Here's how the part is built. I have some questions about the finished solid (model axes, mm). Coordinates: 2 decimals unless noted, no trailing zeros. Write each loop counter-clockwise with the first axis right and the second up, starting at its lowest first coordinate (ties: lowest second). Pieces come first, ordered by that corner, then holes. Notation, with made-up numbers: (82, -29) - (130, -29) arc R14 ccw to (130, -24) - close; hole circle Ø2 at (39.25, 64.5). An arc over 180 degrees is marked (long way). Answer in a Markdown table with one row per item. Add a question column.
Item 1: Imagine slicing it at D-D (x = 134.5). Please give me the cut outline in (y, z).
Item 2: If I drill on probe 1 along Y at (x, z) = (118.5, 63); probe 2 along X at (y, z) = (-15, 8.5); probe 3 along Z at (x, y) = (-47, -74.5), over which ranges is the centre line in solid material (lowest first)? Write a range as from..to.
Item 3: Imagine slicing it at C-C (z = 71.5). Please give me the cut outline in (x, y).
Item 4: Imagine slicing it at B-B (y = -29.5). Please give me the cut outline in (x, z).
Item 5: I'm going to push flat-ended pins straight in: pin 1 (4 mm diameter, centred on y = -114, z = -4.5, fed in from -X); pin 2 (10 mm diameter, centred on y = -34.5, z = 7, fed in from -X); pin 3 (3 mm diameter, centred on x = -71.5, z = -162.5, fed in from +Y). Where does each tip first touch, or does it pass through?
Item 6: Imagine slicing it at A-A (x = 2). Please give me the cut outline in (y, z).
from build123d import *

# Parameters (mm, degrees)
F1_DEPTH = 139.7
F3_DEPTH = 254


with BuildPart() as f1:
    # F0 (on Front) → F1 (new body)
    with BuildSketch(Plane.XZ):
        Polygon((-101.6, 100.334205), (-152.4, 12.7), (-101.6, -140.965795), (-93.98, -204.465795), (0, -204.465795), (0, 100.334205), align=None)
        Polygon((101.6, 100.334205), (0, 100.334205), (0, -204.465795), (93.98, -204.465795), (101.6, -140.965795), (152.4, 12.7), align=None)
    extrude(amount=F1_DEPTH)

    # F2 (on Right) → F3 (cut, symmetric)
    with BuildSketch(Plane.YZ):
        Polygon((11.297926, 100.633033), (-45.92489, 100.633033), (0, 12.690174), (-88.975355, -204.561785), (-139.714777, -28.677866), (-46.015032, 100.633033), (-152.156293, 100.633033), (-152.156293, -218.677998), (11.297926, -218.677998), align=None)
    extrude(amount=F3_DEPTH, both=True, mode=Mode.SUBTRACT)


solid = f1.part
Here are the results:
| question | item | result |
|---|---|---|
| 1 | outline | (-139.7, -28.73) - (-136.03, -41.45) - (-22.17, -41.45) - (0, 12.69) - (-16.13, 43.58) - (-87.36, 43.58) - (-139.7, -28.66) - close |
| 2 | probe 1 | y = -73.28..-26.27 |
| 2 | probe 2 | x = -151.01..151.01 |
| 2 | probe 3 | z = -169.22..61.32 |
| 3 | outline | (-118.31, -67.13) - (118.31, -67.13) - (118.31, -30.71) - (-118.31, -30.71) - close |
| 4 | outline | (-152.4, 12.7) - (-128.58, -59.34) - (128.58, -59.34) - (152.4, 12.7) - (119.66, 69.18) - (-119.66, 69.18) - close |
| 5 | pin 1 | stops at x = -147.38 |
| 5 | pin 2 | stops at x = -152.17 |
| 5 | pin 3 | stops at y = -71.13 |
| 6 | outline | (-139.7, -28.73) - (-89, -204.47) - (-88.94, -204.47) - (0, 12.69) - (-45.77, 100.33) - (-46.23, 100.33) - (-139.7, -28.66) - close |
